Check sheet for the drawn part. Datum: minimum x, y, z corner. Units: mm. A direction names the side the tool comes from. Give positions to 0.01 mm unless a question says otherwise; leave off trailing zeros. Loops run counter-clockwise (first coordinate to the right, second up) from the corner with the lowest first, then second, coordinate; pieces in that order, holes last.
1. Cross-section at C-C, the plane x = 10. Record the cut outline in (y, z).
2. Cross-section at A-A, the plane z = 10. Record the cut outline in (x, y).
3. Cross-section at B-B, the plane y = 52. Record the cut outline in (x, z).
4. Release check for a two-part mould opening along Z. For the marked faces 3, 4 and 5 record: +Z half, -Z half, draft (parallel to the pull), parting line (faces both ways), or undercut.
5. Material ranges on L1, parallel to X at y = 24, z = 11.75; L2, parallel to Y at x = 10, z = 0.45, recorded low to high.
6. Cross-section at D-D, the plane z = 3. Record the cut outline in (x, y).
7. Tool access check on the marked faces 1 and 2. Record the directions out of +Z, -Z, +X, -X, +Y, -Y that give a thin tool (end or side, any length) a straight path to the whole face; none if there is none.
8. Go/stop test with a flat-tipped pin: pin 1 Ø4 at (x, y) = (10, 10.8) entering from -Z (3 decimals). Record where the tip stops, or that it passes through.
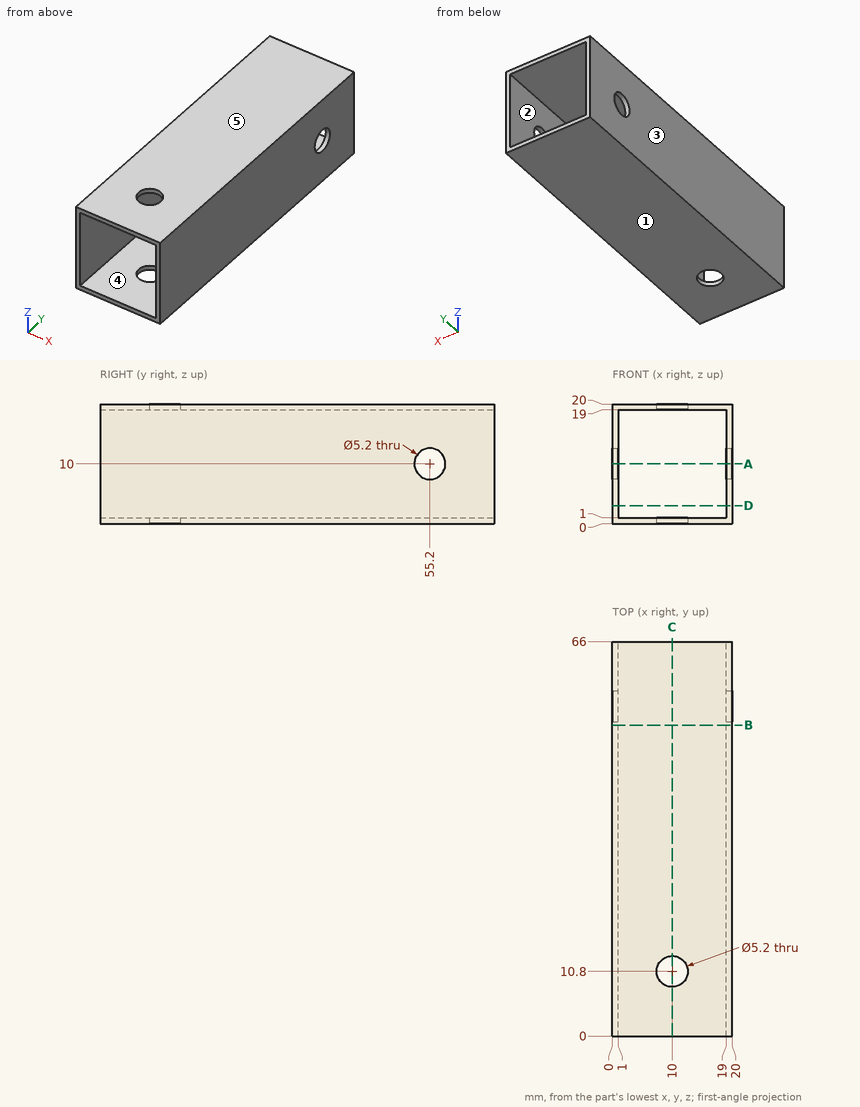
Result:
1. outline: (0, 0) - (8.2, 0) - (8.2, 1) - (0, 1) - close; (0, 19) - (8.2, 19) - (8.2, 20) - (0, 20) - close; (13.4, 0) - (66, 0) - (66, 1) - (13.4, 1) - close; (13.4, 19) - (66, 19) - (66, 20) - (13.4, 20) - close
2. outline: (0, 0) - (1, 0) - (1, 52.6) - (0, 52.6) - close; (0, 57.8) - (1, 57.8) - (1, 66) - (0, 66) - close; (19, 0) - (20, 0) - (20, 52.6) - (19, 52.6) - close; (19, 57.8) - (20, 57.8) - (20, 66) - (19, 66) - close
3. outline: (0, 0) - (20, 0) - (20, 20) - (0, 20) - close; hole (1, 1) - (19, 1) - (19, 19) - (1, 19) - close
4. face 3: draft
4. face 4: undercut
4. face 5: +Z half
5. L1: x = 0 to 1, 19 to 20
5. L2: y = 0 to 8.2, 13.4 to 66
6. outline: (0, 0) - (1, 0) - (1, 66) - (0, 66) - close; (19, 0) - (20, 0) - (20, 66) - (19, 66) - close
7. face 1: -Z, +X, -X, +Y, -Y
7. face 2: +Y, -Y
8. pin 1: passes through
